Solid Edge part; units mm, degrees
sketch "Sketch1" plane through (0, 0, 0) normal (0, 0, 1) x (1, 0, 0)
  circle A0 centre (0, 0) radius 2.45
extrude "Protrusion1" add sketch "Sketch1" along normal blind 8
chamfer "Chamfer_1" distance 0.5 angle 45 2 edges at (-2.45, 0, 8) (-2.45, 0, 0)
sketch "Sketch2" plane through (0, 0, 0) normal (0, 0, -1) x (0, 1, 0)
  line L0 (-1.4, 0) -> (-0.7, 1.2124)
  line L1 (-0.7, 1.2124) -> (0.7, 1.2124)
  line L2 (0.7, 1.2124) -> (1.4, 0)
  line L3 (1.4, 0) -> (0.7, -1.2124)
  line L4 (0.7, -1.2124) -> (-0.7, -1.2124)
  line L5 (-0.7, -1.2124) -> (-1.4, 0)
extrude "ExtrudedCutout_1" cut sketch "Sketch2" against normal blind 1
properties material "Stainless steel"
Geometry check sheet. Reference: the model listing, model coordinates, mm. A direction names the side the tool comes from. Coordinates: 2 decimals unless noted, no trailing zeros. Order: outer loops, then holes, each group sorted by start corner. A loop starts at its lowest first (then second) coordinate and runs counter-clockwise, first axis right, second up. Notation, with made-up numbers: (79, -6.5) -> (85, -6.5) arc R26 cw to (85, 7.5) -> close; hole circle Ø1 at (76.25, 6). An arc over 180 degrees is marked (long way). Use a Markdown table: item, result. Add a question column.
1. Mould release check, pull along Y, two halves, no side actions. Record for faces 3 (the face through (-0.5, 2.4, 4)), 4 (the face through (-0.61, -1.05, 0.49)), 5 (the face through (-1, 1, 0)): pulls with the +Y half, pulls with the -Y half, needs draft (parallel to the pull), parting line crosses it, or undercut.
2. Cross-section at A-A (y = 0). Enter the section's corners in (x, z).
3. Go/stop test with flat-tipped pins: pin 1 Ø2 at (y, z) = (-1.5, 7) entering from +X; pin 2 Ø0.7 at (x, y) = (-0.5, 0.5) entering from -Z. Record where each tip stops, or that it passes through.
4. Set-up check for faces 1 (the face through (0, 0, 8)), 2 (the face through (0.598, -1.055, 0.493)): record each of +Z, -Z, +X, -X, +Y, -Y from which the full face is reachable in a straight line by a thin tool's end or side.
5. Cross-section at B-B (z = 2.75). Enter the section's corners in (x, y), and give its area (3 significant figures).
6. Material ranges on L1, parallel to Z at x = 0.15, y = -0.75; L2, parallel to Y at x = 0.1, z = 4.25; L3, parallel to X at y = 0.75, z = 7, recorded low to high.
Filled sheet:
| question | item | result |
|---|---|---|
| 1 | face 3 | parting line crosses it |
| 1 | face 4 | undercut |
| 1 | face 5 | needs draft |
| 2 | outline | (-2.45, 0.5) -> (-1.95, 0) -> (-1.21, 0) -> (-1.21, 1) -> (1.21, 1) -> (1.21, 0) -> (1.95, 0) -> (2.45, 0.5) -> (2.45, 7.5) -> (1.95, 8) -> (-1.95, 8) -> (-2.45, 7.5) -> close |
| 3 | pin 1 | x = 2.4 |
| 3 | pin 2 | z = 1 |
| 4 | face 1 | +Z, +X, -X, +Y, -Y |
| 4 | face 2 | -Z |
| 5 | outline | circle Ø4.9 at (0, 0) |
| 5 | area | 18.9 mm2 |
| 6 | L1 | 1 to 8 |
| 6 | L2 | -2.45 to 2.45 |
| 6 | L3 | -2.33 to 2.33 |
